from build123d import *


with BuildPart() as f1:
    # F0 (on Front) → F1 (revolve)
    with BuildSketch(Plane.XZ):
        Polygon((-100, 0), (0, 0), (0, 5), (-6, 5), (-6, 10), (-18, 10), (-18, 5), (-28, 5), (-28, 10), (-40, 10), (-40, 5), (-60, 5), (-60, 10), (-72, 10), (-72, 5), (-82, 5), (-82, 10), (-94, 10), (-94, 5), (-100, 5), align=None)
    revolve(axis=Axis((-44.310086, 0, 0), (-1, 0, 0)))


solid = f1.part
Model file for the job. Use its own axes, mm. A direction names the side the tool comes from. Coordinates: 2 decimals unless noted, no trailing zeros. Write each loop counter-clockwise with the first axis right and the second up, starting at its lowest first coordinate (ties: lowest second). Pieces come first, ordered by that corner, then holes. Notation, with made-up numbers: (-12.5, -8) -> (31.5, -8) arc R21 cw to (31.5, 17) -> close; hole circle Ø7 at (10.25, -15). An arc over 180 degrees is marked (long way). One line per item, written item: value. Start each with the question number.
1) Slice it at C-C on x = -22. Write the cut outline in (y, z).
2) Probe probe 1 along X at (y, z) = (-0.25, -7); probe 2 along Z at (x, y) = (-89.5, 4.75); probe 3 along Z at (x, y) = (-16, -3.75). List the from-to ranges inside material, lowest first.
3) Pull direction X, two halves, no side cores. Call faces 1 (the face through (-100, 0, 0)), 2 (the face through (-34.08, -9.76, -2.17)), 3 (the face through (-40, 5, 2)): +X half, -X half, draft (parallel to the pull), parting line (faces both ways), or undercut.
4) Flat gauge pins, fed straight in: pin 1 Ø4 at (x, z) = (-73, 7) entering from -Y; pin 2 Ø2 at (x, y) = (-25.5, 1.5) entering from +Z; pin 3 Ø12 at (x, y) = (-57.5, 6) entering from -Z. Where does each tip first touch, or does it go through?
5) Slice it at B-B on x = -67.5. Write the cut outline in (y, z), then the cut area to 3 significant figures.
6) Which spindle directions (+Z, -Z, +X, -X, +Y, -Y) get a long thin tool onto all of the face, cutting with end or side? Do faces 4 (the face through (-12.08, -9.76, -2.17)), 5 (the face through (-94, 5, 2)), 6 (the face through (-82, 5, -2)), 7 (the face through (-3.04, -4.88, -1.08)). Say none if no direction does.
7) Slice it at A-A on y = 8.25. Write the cut outline in (x, z).
Answers follow:
1. outline: circle Ø10 at (0, 0)
2. probe 1: -94 to -82, -72 to -60, -40 to -28, -18 to -6
2. probe 2: -8.8 to 8.8
2. probe 3: -9.27 to 9.27
3. face 1: -X half
3. face 2: draft
3. face 3: undercut
4. pin 1: y = -8.5
4. pin 2: z = 4.97
4. pin 3: z = -9.99
5. outline: circle Ø20 at (0, 0)
5. area: 314 mm2
6. face 4: +X, -X
6. face 5: -X
6. face 6: none
6. face 7: +X
7. outline: (-94, -5.65) -> (-82, -5.65) -> (-82, 5.65) -> (-94, 5.65) -> close; (-72, -5.65) -> (-60, -5.65) -> (-60, 5.65) -> (-72, 5.65) -> close; (-40, -5.65) -> (-28, -5.65) -> (-28, 5.65) -> (-40, 5.65) -> close; (-18, -5.65) -> (-6, -5.65) -> (-6, 5.65) -> (-18, 5.65) -> close
